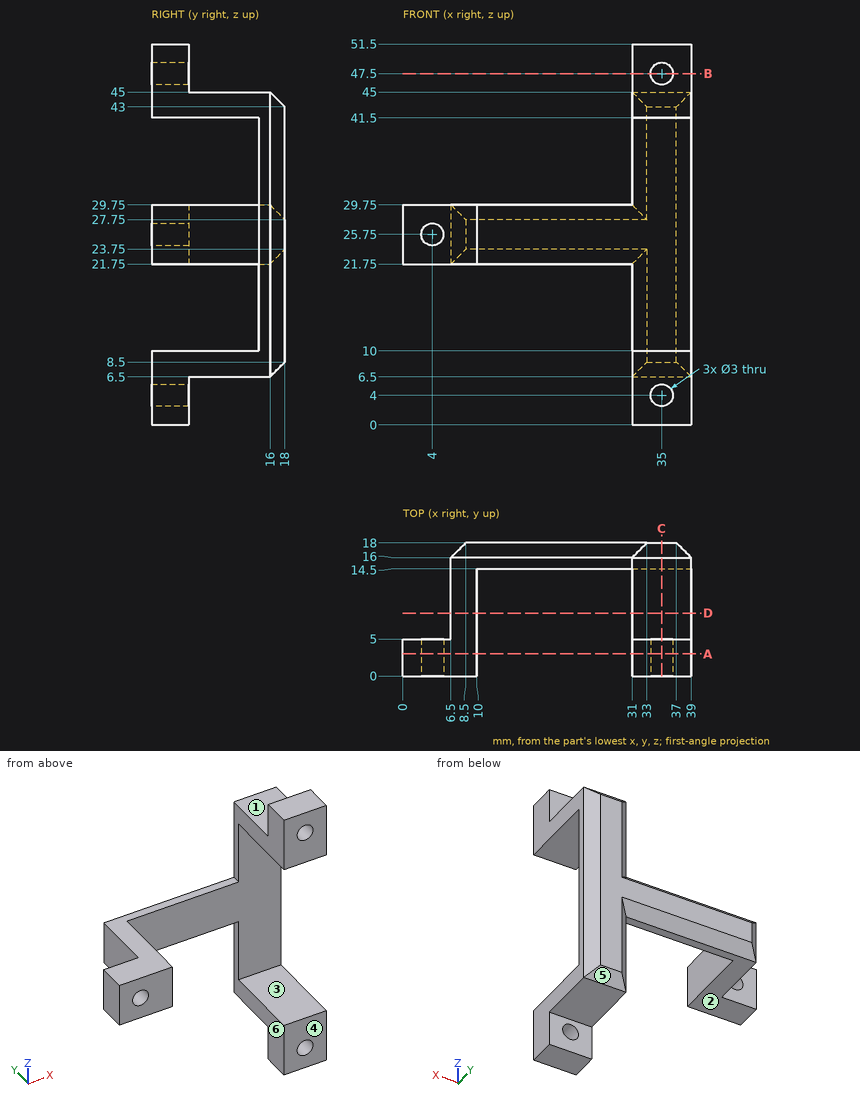
For this review, use the dimensioned drawing (mm, ordinates from the lowest corner) and the shaded views. A direction names the side the tool comes from. Coordinates: 2 decimals unless noted, no trailing zeros. Order: outer loops, then holes, each group sorted by start corner. A loop starts at its lowest first (then second) coordinate and runs counter-clockwise, first axis right, second up. Notation, with made-up numbers: (37.25, -24) - (52.25, -24) arc R16 cw to (52.25, -9) - close; hole circle Ø4 at (16, 74). An arc over 180 degrees is marked (long way). Use one line per item in the form item = value.
Q1. For P1, Ø4, axis at y = 11, z = 27.5, coming from the -X side; P2, Ø8, axis at y = 9.5, z = 11.5, coming from the -X side; P3, Ø7, axis at x = 4.5, z = 25.5, coming from the +Y side, all flat-tipped, find the tip position at first contact; note any pin that passes through.
Checked values:
P1 = 6.5
P2 = 31
P3 = 17.5
Q2. For the marked faces 1, 2 and 3, list the 3-axis set-ups (+Z, -Z, +X, -X, +Y, -Y) from which the entire face can be reached by the end or side of a thin tool; tool diameter is ignored.
Checked values:
face_1 = +Z, +X, -X, +Y
face_2 = -Z, -X, +Y, -Y
face_3 = +X, -X, -Y
Q3. Consider section D-D (y = 8.5). Give the boundary of the cut face in (x, z), then the cut area to 3 significant figures.
Checked values:
outline = (6.5, 21.75) - (10, 21.75) - (10, 29.75) - (6.5, 29.75) - close; (31, 6.5) - (39, 6.5) - (39, 10) - (31, 10) - close; (31, 41.5) - (39, 41.5) - (39, 45) - (31, 45) - close
area = 84.0 mm2
Q4. For probe 1 along X at (y, z) = (1.65, 4); probe 2 along Z at (x, y) = (4, 1.15); probe 3 along Z at (x, y) = (9, 6.75), list the stretches that pass through material, from the lowest coordinate up. Write a range as from..to.
Checked values:
probe_1 = 31..33.5, 36.5..39
probe_2 = 21.75..24.25, 27.25..29.75
probe_3 = 21.75..29.75
Q5. Draft analysis for pull direction Y (two halves, no side actions). For the marked faces 4, 5 and 6, state which applies: +Y half, -Y half, draft (parallel to the pull), parting line (faces both ways), or undercut.
Checked values:
face_4 = -Y half
face_5 = +Y half
face_6 = draft
Q6. Consider section A-A (y = 3). Give the boundary of the cut face in (x, z).
Checked values:
outline = (0, 21.75) - (10, 21.75) - (10, 29.75) - (0, 29.75) - close; (31, 0) - (39, 0) - (39, 10) - (31, 10) - close; (31, 41.5) - (39, 41.5) - (39, 51.5) - (31, 51.5) - close; hole circle Ø3 at (4, 25.75); hole circle Ø3 at (35, 4); hole circle Ø3 at (35, 47.5)
Q7. Consider section B-B (z = 47.5). Give the boundary of the cut face in (x, y).
Checked values:
outline = (31, 0) - (33.5, 0) - (33.5, 5) - (31, 5) - close; (36.5, 0) - (39, 0) - (39, 5) - (36.5, 5) - close
Q8. Consider section C-C (x = 35). Give the boundary of the cut face in (y, z), then the cut area to 3 significant figures.
Checked values:
outline = (0, 0) - (5, 0) - (5, 2.5) - (0, 2.5) - close; (0, 5.5) - (5, 5.5) - (5, 6.5) - (16, 6.5) - (18, 8.5) - (18, 43) - (16, 45) - (5, 45) - (5, 46) - (0, 46) - (0, 41.5) - (14.5, 41.5) - (14.5, 10) - (0, 10) - close; (0, 49) - (5, 49) - (5, 51.5) - (0, 51.5) - close
area = 267 mm2
